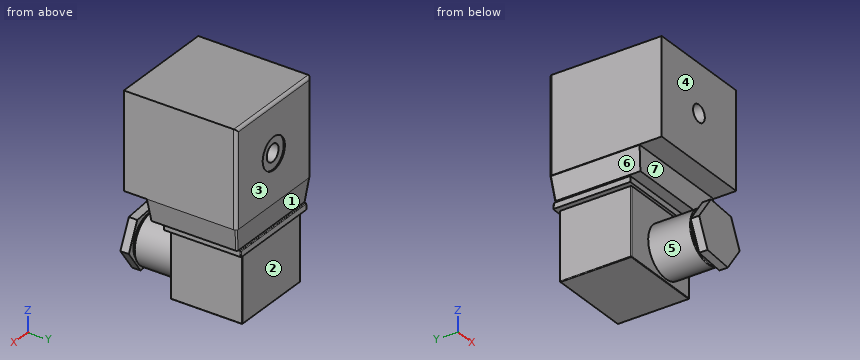
from build123d import *
from OCP.BRepFilletAPI import BRepFilletAPI_MakeChamfer

# Parameters (mm, degrees)
SKETCH2_W                   = 48.26
SKETCH2_H                   = 50.8
BOSS_EXTRUDE1_DEPTH         = 43.18
FILLET1_R                   = 1.27
BOSS_EXTRUDE2_DEPTH         = 10.16
CHAMFER1_SIZE               = 10.16
CHAMFER1_SIZE_2             = 0.888884821
SKETCH4_R                   = 7.183192936
CUT_EXTRUDE1_DEPTH          = 0.508
CHAMFER4_SIZE               = 1.791482124
CHAMFER4_SIZE_2             = 10.16
SKETCH6_W                   = 42.672
SKETCH6_H                   = 34.798230358
BOSS_EXTRUDE3_DEPTH         = 2.54
CHAMFER2_SIZE2              = 2.54
CHAMFER2_SIZE               = 0.222221205
FILLET4_R                   = 0.3175
SKETCH8_W                   = 37.592
SKETCH8_H                   = 32.258230358
BOSS_EXTRUDE4_DEPTH         = 30.48
FILLET5_R                   = 0.3175
FILLET6_R                   = 0.3175
FILLET7_R                   = 0.3175
SKETCH10_R                  = 11.43
BOSS_EXTRUDE5_DEPTH         = 19.05
SKETCH11_R                  = 10.16
BOSS_EXTRUDE6_DEPTH         = 1.27
BOSS_EXTRUDE7_DEPTH         = 3.81
FILLET8_R                   = 0.3175
FILLET2_R                   = 0.635
F_3_64_0_3_DIAMETER_HOLE1_D = 7.62


# Some blends are built 0.0001 mm under size
with BuildPart() as part:
    # Sketch2 → Boss-Extrude1 (new body)
    with BuildSketch(Plane.XY):
        with Locations((24.13, 25.4)):
            Rectangle(SKETCH2_W, SKETCH2_H)
    extrude(amount=BOSS_EXTRUDE1_DEPTH)

    # Fillet1
    fillet1_edges = [part.edges().sort_by_distance(p)[0] for p in [
        (24.13, 50.8, 43.18),
        (0, 50.8, 21.59),
        (48.26, 50.8, 21.59),
    ]]
    fillet(fillet1_edges, radius=FILLET1_R)

    # Sketch3 → Boss-Extrude2 (add)
    with BuildSketch(Plane(origin=(0, 0, 0), x_dir=(-1, 0, 0), z_dir=(0, 0, -1))):
        Polygon((-45.466, 50.546), (-2.794, 50.546), (-0.254, 50.546), (-0.254, 48.006), (-0.254, 10.16), (-48.006, 10.16), (-48.006, 48.006), (-48.006, 50.546), align=None)
    extrude(amount=BOSS_EXTRUDE2_DEPTH)

    # Chamfer1
    chamfer1_edges_1 = [part.edges().sort_by_distance(p)[0] for p in [
        (24.13, 50.546, -10.16),
    ]]
    chamfer1_side_1 = [part.faces().sort_by_distance(p)[0] for p in [
        (24.13, 50.546, -10.142222304),
    ]]
    chamfer1_edges_2 = [part.edges().sort_by_distance(p)[0] for p in [
        (24.13, 10.16, -10.16),
    ]]
    chamfer1_side_2 = [part.faces().sort_by_distance(p)[0] for p in [
        (24.13, 10.16, -10.142222304),
    ]]
    chamfer1 = BRepFilletAPI_MakeChamfer(part.part.solid().wrapped)
    for e in chamfer1_edges_1:
        chamfer1.Add(CHAMFER1_SIZE - 0.0001, CHAMFER1_SIZE_2 - 0.0001, e.wrapped, chamfer1_side_1[0].wrapped)
    for e in chamfer1_edges_2:
        chamfer1.Add(CHAMFER1_SIZE - 0.0001, CHAMFER1_SIZE_2 - 0.0001, e.wrapped, chamfer1_side_2[0].wrapped)
    add(Compound.cast(chamfer1.Shape()), mode=Mode.REPLACE)  # a hair under: the kernel refuses the full size

    # Sketch4 → Cut-Extrude1 (cut)
    with BuildSketch(Plane(origin=(0, 50.8, 0), x_dir=(1, 0, 0), z_dir=(0, 1, 0))):
        with Locations(Location((24.13, -21.59, 0), (0, 0, 270))):
            Circle(SKETCH4_R)
    extrude(amount=-CUT_EXTRUDE1_DEPTH, mode=Mode.SUBTRACT)

    # Chamfer4
    chamfer4_edges_1 = [part.edges().sort_by_distance(p)[0] for p in [
        (48.006, 30.353, -10.16),
    ]]
    chamfer4_side_1 = [part.faces().sort_by_distance(p)[0] for p in [
        (47.970170358, 30.353, -10.16),
    ]]
    chamfer4_edges_2 = [part.edges().sort_by_distance(p)[0] for p in [
        (0.254, 30.353, -10.16),
    ]]
    chamfer4_side_2 = [part.faces().sort_by_distance(p)[0] for p in [
        (0.254, 30.353, -10.124170358),
    ]]
    chamfer4 = BRepFilletAPI_MakeChamfer(part.part.solid().wrapped)
    for e in chamfer4_edges_1:
        chamfer4.Add(CHAMFER4_SIZE - 0.0001, CHAMFER4_SIZE_2 - 0.0001, e.wrapped, chamfer4_side_1[0].wrapped)
    for e in chamfer4_edges_2:
        chamfer4.Add(CHAMFER4_SIZE_2 - 0.0001, CHAMFER4_SIZE - 0.0001, e.wrapped, chamfer4_side_2[0].wrapped)
    add(Compound.cast(chamfer4.Shape()), mode=Mode.REPLACE)  # a hair under: the kernel refuses the full size

    # Sketch6 → Boss-Extrude3 (add)
    with BuildSketch(Plane(origin=(0, 0, -10.16), x_dir=(-1, 0, 0), z_dir=(0, 0, -1))):
        with Locations((-24.13, 33.528)):
            Rectangle(SKETCH6_W, SKETCH6_H)
    extrude(amount=BOSS_EXTRUDE3_DEPTH)

    # Chamfer2
    chamfer2_edges = [part.edges().sort_by_distance(p)[0] for p in [
        (24.13, 50.927115179, -10.16),
    ]]
    chamfer2_side = [part.faces().sort_by_distance(p)[0] for p in [
        (24.13, 50.922670754, -10.16),
    ]]
    chamfer(chamfer2_edges, length=CHAMFER2_SIZE - 0.0001, length2=CHAMFER2_SIZE2 - 0.0001, reference=chamfer2_side[0])  # a hair under: the kernel refuses the full size

    # Fillet4
    # the kernel refuses this fillet: 0.3175 mm, written as the material it takes off along each edge
    with BuildSketch(Plane(origin=(45.466, 50.635842296, -9.369267992), x_dir=(-1, 0, 0), z_dir=(0, 0.08712022396653547, -0.9961978049443899)), Plane(origin=(2.794, 50.635842296, -9.369267992), x_dir=(0, -0.9961978049443899, -0.08712022396653547), z_dir=(0, 0.08712022396653547, -0.9961978049443899))) as fillet4_piece_1:
        with BuildLine():
            CenterArc((FILLET4_R, -FILLET4_R), FILLET4_R, 90, 90)
            Line((0, -FILLET4_R), (0, 0))
            Line((0, 0), (FILLET4_R, 0))
        make_face()
    extrude(amount=4.137094054, mode=Mode.SUBTRACT)
    with BuildSketch(Plane(origin=(46.193363902, 50.704993974, -10.16), x_dir=(0, -1, 0), z_dir=(-1, 0, 0))) as fillet4_piece_2:
        with BuildLine():
            CenterArc((FILLET4_R * 0.916363970592, -FILLET4_R), FILLET4_R, 90, 85.002042847)
            Line((-FILLET4_R * 0.0798338343528, -FILLET4_R * 0.912879776033), (0, 0))
            Line((0, 0), (FILLET4_R * 0.916363970592, 0))
        make_face()
    extrude(amount=44.126727803, mode=Mode.SUBTRACT)

    # Sketch8 → Boss-Extrude4 (add)
    with BuildSketch(Plane(origin=(0, 0, -12.7), x_dir=(-1, 0, 0), z_dir=(0, 0, -1))):
        with Locations((-24.13, 33.528)):
            Rectangle(SKETCH8_W, SKETCH8_H)
    extrude(amount=BOSS_EXTRUDE4_DEPTH)

    # Fillet5
    fillet5_edges = [part.edges().sort_by_distance(p)[0] for p in [
        (42.926, 49.657115179, -27.94),
        (5.334, 49.657115179, -27.94),
        (24.13, 49.657115179, -43.18),
    ]]
    fillet(fillet5_edges, radius=FILLET5_R)

    # Fillet6
    # the kernel refuses this fillet: 0.3175 mm, written as the material it takes off along each edge
    with BuildSketch(Plane(origin=(42.6085, 17.716384821, -42.8625), x_dir=(0, -1, 0), z_dir=(1, 0, 0))) as fillet6_piece_1_section:
        Polygon((0, 0), (FILLET6_R * 1.02, 0), (FILLET6_R * 1.02, FILLET6_R * 1.02), (0, FILLET6_R * 1.02), align=None)
    fillet6_piece_1 = extrude(amount=FILLET6_R * 1.02, mode=Mode.PRIVATE)
    fillet6_piece_1 = fillet6_piece_1 - Plane(origin=(42.6085, 17.716384821, -42.8625), x_dir=(0, 0.7071067811865475, 0.7071067811865475), z_dir=(1, 0, 0)) * Sphere(FILLET6_R, mode=Mode.PRIVATE)
    add(fillet6_piece_1, mode=Mode.SUBTRACT)
    with BuildSketch(Plane(origin=(42.926, 17.398884821, -12.7), x_dir=(0, 1, 0), z_dir=(0, 0, -1))) as fillet6_piece_2:
        with BuildLine():
            CenterArc((FILLET6_R, -FILLET6_R), FILLET6_R, 90, 90)
            Line((0, -FILLET6_R), (0, 0))
            Line((0, 0), (FILLET6_R, 0))
        make_face()
    extrude(amount=30.1625, mode=Mode.SUBTRACT)
    with BuildSketch(Plane(origin=(4.54025, 17.398884821, -43.18), x_dir=(0, 0, 1), z_dir=(1, 0, 0))) as fillet6_piece_3:
        with BuildLine():
            CenterArc((FILLET6_R, -FILLET6_R), FILLET6_R, 90, 90)
            Line((0, -FILLET6_R), (0, 0))
            Line((0, 0), (FILLET6_R, 0))
        make_face()
    extrude(amount=38.06825, mode=Mode.SUBTRACT)
    with BuildSketch(Plane(origin=(5.334, 50.133365179, -43.18), x_dir=(0, 0, 1), z_dir=(0, -1, 0))) as fillet6_piece_4:
        with BuildLine():
            CenterArc((FILLET6_R, -FILLET6_R), FILLET6_R, 90, 90)
            Line((0, -FILLET6_R), (0, 0))
            Line((0, 0), (FILLET6_R, 0))
        make_face()
    extrude(amount=33.528230357, mode=Mode.SUBTRACT)
    with BuildSketch(Plane(origin=(42.926, 17.716384821, -43.18), x_dir=(0, 0, 1), z_dir=(0, 1, 0))) as fillet6_piece_5:
        with BuildLine():
            CenterArc((FILLET6_R, -FILLET6_R), FILLET6_R, 90, 90)
            Line((0, -FILLET6_R), (0, 0))
            Line((0, 0), (FILLET6_R, 0))
        make_face()
    extrude(amount=32.416980357, mode=Mode.SUBTRACT)

    # Fillet7
    # the kernel refuses this fillet: 0.3175 mm, written as the material it takes off along each edge
    with BuildSketch(Plane(origin=(5.6515, 17.716384821, -42.8625), x_dir=(-1, 0, 0), z_dir=(0, -1, 0))) as fillet7_piece_1_section:
        Polygon((0, 0), (FILLET7_R, 0), (FILLET7_R, FILLET7_R), (0, FILLET7_R), align=None)
    fillet7_piece_1 = extrude(amount=FILLET7_R, mode=Mode.PRIVATE)
    fillet7_piece_1 = fillet7_piece_1 - Plane(origin=(5.6515, 17.716384821, -42.8625), x_dir=(0.7071067811865475, 0, 0.7071067811865475), z_dir=(0, -1, 0)) * Sphere(FILLET7_R, mode=Mode.PRIVATE)
    add(fillet7_piece_1, mode=Mode.SUBTRACT)
    with BuildSketch(Plane(origin=(5.334, 17.398884821, -12.7), x_dir=(1, 0, 0), z_dir=(0, 0, -1))) as fillet7_piece_2:
        with BuildLine():
            CenterArc((FILLET7_R, -FILLET7_R), FILLET7_R, 90, 90)
            Line((0, -FILLET7_R), (0, 0))
            Line((0, 0), (FILLET7_R, 0))
        make_face()
    extrude(amount=30.1625, mode=Mode.SUBTRACT)

    # Sketch10 → Boss-Extrude5 (add)
    with BuildSketch(Plane.XZ.offset(-17.398884821)):
        with Locations(Location((27.686, -30.48, 0), (0, 0, 90))):
            Circle(SKETCH10_R)
    extrude(amount=BOSS_EXTRUDE5_DEPTH)

    # Sketch11 → Boss-Extrude6 (add)
    with BuildSketch(Plane.XZ.offset(1.651115179)):
        with Locations(Location((27.686, -30.48, 0), (0, 0, 270))):
            Circle(SKETCH11_R)
    extrude(amount=BOSS_EXTRUDE6_DEPTH)

    # Sketch12 → Boss-Extrude7 (add)
    with BuildSketch(Plane.XZ.offset(2.921115179)):
        Polygon((33.181274645, -42.479798189), (40.825767394, -31.720851652), (35.33049275, -19.721053462), (22.190725355, -18.480201811), (14.546232606, -29.239148348), (20.04150725, -41.238946538), align=None)
    extrude(amount=BOSS_EXTRUDE7_DEPTH)

    # Fillet8
    fillet8_edges = [part.edges().sort_by_distance(p)[0] for p in [
        (27.686, -1.651115179, -41.91),
    ]]
    fillet(fillet8_edges, radius=FILLET8_R)

    # Fillet2
    # the kernel refuses this fillet: 0.635 mm, written as the material it takes off along each edge
    with BuildSketch(Plane(origin=(45.944105867, 49.523002068, -11.694220381), x_dir=(0.01490405395374314, -0.9963095509323676, 0.08452897666887954), z_dir=(0.17299962328390456, 0.08583285338927087, 0.9811747304240377))) as fillet2_piece_1_section:
        with BuildLine():
            CenterArc((FILLET2_R * 0.984980559667, -FILLET2_R), FILLET2_R, 90, 89.132954612)
            Line((-FILLET2_R * 0.0149049417488, -FILLET2_R * 0.984867780788), (0, 0))
            Line((0, 0), (FILLET2_R * 0.984980559667, 0))
        make_face()
    fillet2_piece_1 = extrude(amount=13.48214579, mode=Mode.PRIVATE)
    fillet2_piece_1 = split(fillet2_piece_1, bisect_by=Plane(origin=(46.959597239, 49.956662585, -10.16), z_dir=(0, 0, 1)), keep=Keep.TOP, mode=Mode.PRIVATE)
    fillet2_piece_1 = split(fillet2_piece_1, bisect_by=Plane(origin=(46.959597239, 49.956662585, 0), z_dir=(0, 0, -1)), keep=Keep.TOP, mode=Mode.PRIVATE)
    add(fillet2_piece_1, mode=Mode.SUBTRACT)
    with BuildSketch(Plane(origin=(-0.016512009, 50.680213111, 1.534120381), x_dir=(-0.014904053953745064, -0.9963095509323676, 0.0845289766688792), z_dir=(0.17299962328390434, -0.08583285338927088, -0.9811747304240378))) as fillet2_piece_2_section:
        with BuildLine():
            CenterArc((FILLET2_R * 0.984980559667, -FILLET2_R), FILLET2_R, 90, 89.132954612)
            Line((-FILLET2_R * 0.0149049417488, -FILLET2_R * 0.984867780788), (0, 0))
            Line((0, 0), (FILLET2_R * 0.984980559667, 0))
        make_face()
    fillet2_piece_2 = extrude(amount=13.48214579, mode=Mode.PRIVATE)
    fillet2_piece_2 = split(fillet2_piece_2, bisect_by=Plane(origin=(0.354174002, 50.466816982, -10.16), z_dir=(0, 0, 1)), keep=Keep.TOP, mode=Mode.PRIVATE)
    fillet2_piece_2 = split(fillet2_piece_2, bisect_by=Plane(origin=(0.354174002, 50.466816982, 0), z_dir=(0, 0, -1)), keep=Keep.TOP, mode=Mode.PRIVATE)
    add(fillet2_piece_2, mode=Mode.SUBTRACT)

    # 3/64 (0.3) Diameter Hole1 (through all)
    with Locations(Plane(origin=(0, 50.292, 0), x_dir=(1, 0, 0), z_dir=(0, 1, 0))):
        with Locations((24.13, -21.59)):
            Hole(F_3_64_0_3_DIAMETER_HOLE1_D / 2)


solid = part.part
For this review, take the finished solid that the model builds, in its own axes (mm). Face numbers are marked on the shaded views. A direction names the side the tool comes from. Give positions to 0.01 mm unless a question says otherwise; leave off trailing zeros. Loops run counter-clockwise (first coordinate to the right, second up) from the corner with the lowest first, then second, coordinate; pieces in that order, holes last. Notation, with made-up numbers: (-20, -4) -> (7, -4) arc R18 cw to (7, 4) -> close; hole circle Ø6 at (-30, 85.5). An arc over 180 degrees is marked (long way). One line per question, with ' | ' between items.
1) Insertion check: pin 1 Ø0.8 at (x, z) = (19, -11) entering from -Y; pin 2 Ø3 at (x, z) = (21, -10) entering from +Y; pin 3 Ø1 at (x, z) = (11, 8.5) entering from -Y. Each pin has a flat end and moves straight along its axis. Give the tip position at first contact, or say it passes through.
Resolved:
pin 1: stops at y = 16.13 | pin 2: stops at y = 50.82 | pin 3: stops at y = 0
2) We need section A-A (z = 21.59). Write out the cut boundary in (x, y).
Resolved:
outline: (0, 0) -> (20.32, 0) -> (20.32, 50.29) -> (16.95, 50.29) -> (16.95, 50.8) -> (1.27, 50.8) arc R1.27 ccw to (0, 49.53) -> close; (27.94, 0) -> (48.26, 0) -> (48.26, 49.53) arc R1.27 ccw to (46.99, 50.8) -> (31.31, 50.8) -> (31.31, 50.29) -> (27.94, 50.29) -> close
3) For the marked faces 1, 2, 3 and 4, list the 3-axis set-ups (+Z, -Z, +X, -X, +Y, -Y) from which the entire face can be reached by the end or side of a thin tool; tool diameter is ignored.
Resolved:
face 1: +X, -X, +Y | face 2: -Z, +X, -X, +Y | face 3: +Z, +X, -X, +Y | face 4: +Z, +X, -X, -Y
4) We need section D-D (y = 1.5). Write out the cut boundary in (x, z).
Resolved:
outline: (0, 0) -> (48.26, 0) -> (48.26, 43.18) -> (0, 43.18) -> close; circle Ø22.86 at (27.69, -30.48); hole circle Ø7.62 at (24.13, 21.59)
5) The part is to be moulded in two halves that separate along Y. For the marked faces 5, 6 and 7, say which applies: +Y half, -Y half, draft (parallel to the pull), parting line (faces both ways), or undercut.
Resolved:
face 5: undercut | face 6: draft | face 7: -Y half
6) To check wall thickness, follow probe 1 along Z at (x, y) = (24.5, 43); probe 2 along Z at (x, y) = (24, 16); probe 3 along X at (y, z) = (1, 22). State the ranges of each line that lie inside material, in increasing order.
Resolved:
probe 1: z = -43.18 to 17.8, 25.38 to 43.18 | probe 2: z = -41.3 to -19.66, -10.16 to 17.78, 25.4 to 43.18 | probe 3: x = 0 to 20.34, 27.92 to 48.26
